CAD build for the part. Positions are in the model's coordinates, mm. Coordinates: 2 decimals unless noted, no trailing zeros. One line per question, with ' | ' between items. Start each with the question number.
1. Probe line 1 (Y direction, x = -9.75, z = -896.5); line 2 (X direction, y = 13, z = -355); line 3 (X direction, y = -12.25, z = -124.5). List the from-to ranges inside material, lowest first.
2. Band-saw the part on A-A, the plane z = -1051.5. Give the number of separate pieces and of enclosed holes in the cut face, then the cut area to 3 significant figures.
3. Flat gauge pins, fed straight in: P1, Ø1.5, axis at x = -10.5, y = 4.5, coming from the -Z side; P2, Ø6, axis at x = -0.5, z = -505.5, coming from the +Y side; P3, Ø1, axis at y = -2.5, z = -287.5, coming from the -X side; P4, Ø0.6, axis at x = 14.5, z = -722.5, coming from the +Y side. Where does each tip first touch, or does it go through?
Autodesk Inventor part; units mm, degrees
ref_plane "YZ Plane" through (0, 0, 0) normal (1, 0, 0) x (0, 1, 0)
ref_plane "XZ Plane" through (0, 0, 0) normal (0, 1, 0) x (-1, 0, 0)
ref_plane "XY Plane" through (0, 0, 0) normal (0, 0, 1) x (1, 0, 0)
sketch "Sketch1" plane through (0, 0, 0) normal (0, 0, 1) x (1, 0, 0)
  circle A0 centre (-11.375, 11.375) radius 2.1
  circle A1 centre (-11.375, -11.375) radius 2.1
  line L0 (-15, 4.1) -> (-12.9, 4.1)
  line L1 (-12.9, 4.1) -> (-12.9, 8.28)
  line L2 (-12.9, 8.28) -> (-9.85, 8.28)
  line L3 (-9.85, 8.28) -> (-5.8, 4.23)
  line L4 (-5.8, 4.23) -> (-5.8, -4.23)
  line L5 (-5.8, -4.23) -> (-9.85, -8.28)
  line L6 (-9.85, -8.28) -> (-12.9, -8.28)
  line L7 (-12.9, -8.28) -> (-12.9, -4.1)
  line L8 (-12.9, -4.1) -> (-15, -4.1)
  line L9 (-15, -4.1) -> (-15, -13)
  arc A2 (-15, -13) -> (-13, -15) centre (-13, -13) ccw
  line L10 (-13, -15) -> (-4.1, -15)
  line L11 (-4.1, -15) -> (-4.1, -12.9)
  line L12 (-4.1, -12.9) -> (-8.28, -12.9)
  line L13 (-8.28, -12.9) -> (-8.28, -9.85)
  line L14 (-8.28, -9.85) -> (-3.719, -5.289)
  line L15 (-3.719, -5.289) -> (3.719, -5.289)
  line L16 (3.719, -5.289) -> (8.28, -9.85)
  line L17 (8.28, -9.85) -> (8.28, -12.9)
  line L18 (8.28, -12.9) -> (4.1, -12.9)
  line L19 (4.1, -12.9) -> (4.1, -15)
  line L20 (4.1, -15) -> (13, -15)
  arc A3 (13, -15) -> (15, -13) centre (13, -13) ccw
  line L21 (15, -13) -> (15, -4.1)
  line L22 (15, -4.1) -> (12.9, -4.1)
  line L23 (12.9, -4.1) -> (12.9, -8.28)
  line L24 (12.9, -8.28) -> (9.85, -8.28)
  line L25 (9.85, -8.28) -> (5.8, -4.23)
  line L26 (5.8, -4.23) -> (5.8, 4.23)
  line L27 (5.8, 4.23) -> (9.85, 8.28)
  line L28 (9.85, 8.28) -> (12.9, 8.28)
  line L29 (12.9, 8.28) -> (12.9, 4.1)
  line L30 (12.9, 4.1) -> (15, 4.1)
  line L31 (15, 4.1) -> (15, 13)
  arc A4 (15, 13) -> (13, 15) centre (13, 13) ccw
  line L32 (13, 15) -> (4.1, 15)
  line L33 (4.1, 15) -> (4.1, 12.9)
  line L34 (4.1, 12.9) -> (8.28, 12.9)
  line L35 (8.28, 12.9) -> (8.28, 9.85)
  line L36 (8.28, 9.85) -> (3.719, 5.289)
  line L37 (3.719, 5.289) -> (-3.719, 5.289)
  line L38 (-3.719, 5.289) -> (-8.28, 9.85)
  line L39 (-8.28, 9.85) -> (-8.28, 12.9)
  line L40 (-8.28, 12.9) -> (-4.1, 12.9)
  line L41 (-4.1, 12.9) -> (-4.1, 15)
  line L42 (-4.1, 15) -> (-13, 15)
  arc A5 (-13, 15) -> (-15, 13) centre (-13, 13) ccw
  line L43 (-15, 13) -> (-15, 4.1)
  circle A6 centre (0, 0) radius 3.4
  circle A7 centre (11.375, 11.375) radius 2.1
  circle A8 centre (11.375, -11.375) radius 2.1
extrude "Extrusion1" add sketch "Sketch1" against normal blind 1350
sketch "Sketch2" plane through (0, 0, 0) normal (0, 0, 1) x (1, 0, 0)
  point P0 (0, 0)
properties part number "Metal_Profile 135cm" material "Aluminum 6061-AHC"
Filled in:
1) line 1: y = -15 to -12.71, -10.04 to -8.18, 8.18 to 10.04, 12.71 to 15 | line 2: x = -15 to -12.71, -10.04 to -4.1, 4.1 to 10.04, 12.71 to 15 | line 3: x = -15 to -13.28, -9.47 to -8.28, 8.28 to 9.47, 13.28 to 15
2) separate pieces: 1 | enclosed holes: 5 | area: 323 mm²
3) P1: passes through | P2: stops at y = 5.29 | P3: stops at x = -5.8 | P4: stops at y = 14.6
